Could you check a few things on this model? Use its own coordinates, in mm. Face numbers are marked on the shaded views. A direction names the side the tool comes from. Give positions to 0.01 mm unless a question says otherwise; leave off trailing zeros. Loops run counter-clockwise (first coordinate to the right, second up) from the corner with the lowest first, then second, coordinate; pieces in that order, holes last. Notation, with made-up numbers: (-33, 86) - (-6, 86) arc R11 cw to (-6, 100) - close; hole circle Ø11 at (56.25, 41.5). An arc over 180 degrees is marked (long way). Answer in a Markdown table with one row per item. Add a question column.
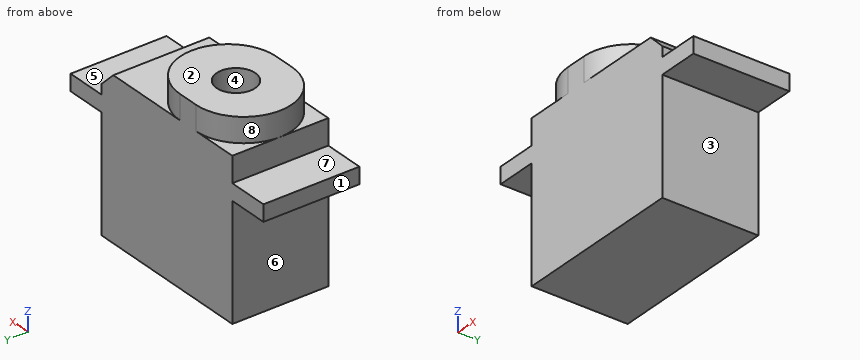
```python
from build123d import *

# Parameters (mm, degrees)
F0_W     = 5.08
F0_H     = 2.032
F1_DEPTH = 11.938
F2_SIZE  = 1.905
F3_R     = 2.4007388602
F4_DEPTH = 3.048


with BuildPart() as f1:
    # F0 (on Front) → F1 (new body)
    with BuildSketch(Plane.XZ):
        with Locations((-2.54, -4.191)):
            Rectangle(F0_W, F0_H)
        with Locations((23.876, -4.191)):
            Rectangle(F0_W, F0_H)
        Polygon((14.478, 0), (0, 0), (0, -3.175), (0, -5.207), (0, -19.431), (21.336, -19.431), (21.336, -5.207), (21.336, -3.175), (21.336, 0), align=None)
    extrude(amount=F1_DEPTH)

    # F2
    f2_edges = [f1.edges().sort_by_distance(p)[0] for p in [
        (21.336, -5.969, 0),
    ]]
    chamfer(f2_edges, length=F2_SIZE)

    # F3 (on face) → F4 (join)
    with BuildSketch(Plane.XY):
        with BuildLine():
            ThreePointArc((7.239, -0.1366710484), (6.6076663792, -0.0342661175), (5.969, 0))
            ThreePointArc((5.969, 0), (0, -5.969), (5.969, -11.938))
            ThreePointArc((5.969, -11.938), (6.6076663792, -11.9037338825), (7.239, -11.8013289516))
            ThreePointArc((7.239, -11.8013289516), (2.54, -5.969), (7.239, -0.1366710484))
        make_face()
        with BuildLine():
            Line((8.509, 0), (5.969, 0))
            ThreePointArc((5.969, 0), (6.6076663792, -0.0342661175), (7.239, -0.1366710484))
            ThreePointArc((7.239, -0.1366710484), (7.8703336208, -0.0342661175), (8.509, 0))
        make_face()
        with BuildLine():
            ThreePointArc((7.239, -11.8013289516), (6.6076663792, -11.9037338825), (5.969, -11.938))
            Line((5.969, -11.938), (8.509, -11.938))
            ThreePointArc((8.509, -11.938), (7.8703336208, -11.9037338825), (7.239, -11.8013289516))
        make_face()
        with BuildLine():
            ThreePointArc((8.509, 0), (7.8703336208, -0.0342661175), (7.239, -0.1366710484))
            ThreePointArc((7.239, -0.1366710484), (10.6170959005, -2.2241147548), (11.938, -5.969))
            ThreePointArc((11.938, -5.969), (10.6170959005, -9.7138852452), (7.239, -11.8013289516))
            ThreePointArc((7.239, -11.8013289516), (7.8703336208, -11.9037338825), (8.509, -11.938))
            ThreePointArc((8.509, -11.938), (12.7297203769, -10.1897203769), (14.478, -5.969))
            ThreePointArc((14.478, -5.969), (12.7297203769, -1.7482796231), (8.509, 0))
        make_face()
        with BuildLine():
            ThreePointArc((7.239, -11.8013289516), (10.6170959005, -9.7138852452), (11.938, -5.969))
            ThreePointArc((11.938, -5.969), (10.6170959005, -2.2241147548), (7.239, -0.1366710484))
            ThreePointArc((7.239, -0.1366710484), (2.54, -5.969), (7.239, -11.8013289516))
        make_face()
        with Locations((7.239, -5.969)):
            Circle(F3_R, mode=Mode.SUBTRACT)
    extrude(amount=F4_DEPTH)


solid = f1.part
```
(1) For pin 1 Ø1.6 at (y, z) = (-3.5, -1) entering from -X; pin 2 Ø3 at (y, z) = (-3, -0.5) entering from +X; pin 3 Ø1.5 at (x, y) = (23, -7) entering from +Z (3 decimals), each with a flat end and sliding along its axis, tell me the tip position at first contact or that it passes through.
(2) On a 3-axis mill with a long thin cutter (end or side, diameter ignored), from which of +Z, -Z, +X, -X, +Y, -Y can I reach the whole of each face in a straight line? I mean the marked faces 5, 6, 7 and 8. Say none if no direction works.
(3) I want a section at D-D on y = -3. Please give me the cut outline in (x, z) (3 decimals), then the cut area to 3 significant figures.
(4) Please list where these lines run through material, in increasing order: line 1 (X direction, y = -7, z = 1.75); line 2 (X direction, y = -10.25, z = -9.75); line 3 (Z direction, x = -0.5, y = -5.5) (3 decimals).
(5) I want a section at A-A on x = 0.5. Please give me the cut outline in (y, z), then the cut area to 3 significant figures.
(6) We'd pull the mould along X, two halves only. Please class the marked faces 1, 2, 3 and 4: pulls with the +X half, pulls with the -X half, needs draft (parallel to the pull), parting line crosses it, or undercut.
(7) I want a section at B-B on y = -7.5. Please give me the cut outline in (x, z) (3 decimals).
(8) I want a section at C-C on z = -10.25. Please give me the cut outline in (x, y), then the cut area to 3 significant figures.
Reported:
| question | item | result |
|---|---|---|
| 1 | pin 1 | x = 0 |
| 1 | pin 2 | x = 21.34 |
| 1 | pin 3 | z = -3.175 |
| 2 | face 5 | +Z, +X, +Y, -Y |
| 2 | face 6 | -Z, -X, +Y, -Y |
| 2 | face 7 | +Z, -X, +Y, -Y |
| 2 | face 8 | +Z, -X |
| 3 | outline | (-5.08, -5.207) - (0, -5.207) - (0, -19.431) - (21.336, -19.431) - (21.336, -5.207) - (26.416, -5.207) - (26.416, -3.175) - (21.336, -3.175) - (21.336, -1.905) - (19.431, 0) - (13.687, 0) - (13.687, 3.048) - (0.791, 3.048) - (0.791, 0) - (0, 0) - (0, -3.175) - (-5.08, -3.175) - close |
| 3 | area | 473 mm² |
| 4 | line 1 | 0.09 to 5.07, 9.41 to 14.39 |
| 4 | line 2 | 0 to 21.34 |
| 4 | line 3 | -5.207 to -3.175 |
| 5 | outline | (-11.94, -19.43) - (0, -19.43) - (0, 0) - (-3.58, 0) - (-3.58, 3.05) - (-8.36, 3.05) - (-8.36, 0) - (-11.94, 0) - close |
| 5 | area | 247 mm² |
| 6 | face 1 | pulls with the -X half |
| 6 | face 2 | needs draft |
| 6 | face 3 | pulls with the +X half |
| 6 | face 4 | undercut |
| 7 | outline | (-5.08, -5.207) - (0, -5.207) - (0, -19.431) - (21.336, -19.431) - (21.336, -5.207) - (26.416, -5.207) - (26.416, -3.175) - (21.336, -3.175) - (21.336, -1.905) - (19.431, 0) - (14.278, 0) - (14.278, 3.048) - (9.088, 3.048) - (9.088, 0) - (5.39, 0) - (5.39, 3.048) - (0.2, 3.048) - (0.2, 0) - (0, 0) - (0, -3.175) - (-5.08, -3.175) - close |
| 8 | outline | (0, -11.94) - (21.34, -11.94) - (21.34, 0) - (0, 0) - close |
| 8 | area | 255 mm² |
